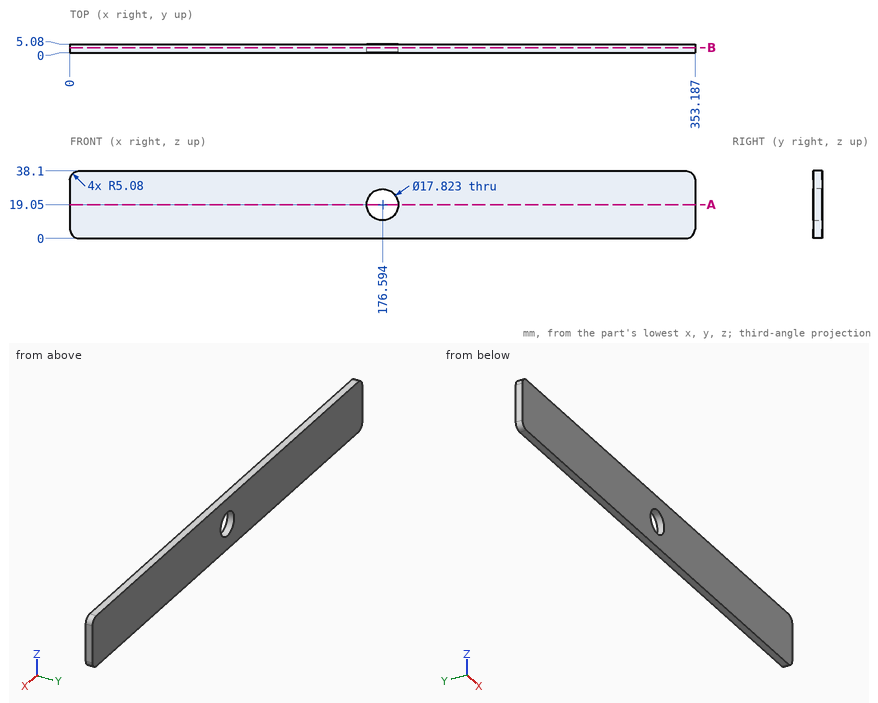
Check sheet for the drawn part. Datum: minimum x, y, z corner. Units: mm. Round coordinates to 2 decimals unless told otherwise and drop trailing zeros. Order: outer loops, then holes, each group sorted by start corner. A loop starts at its lowest first (then second) coordinate and runs counter-clockwise, first axis right, second up.
1. Thickness scan on L1, parallel to X at y = 2.95, z = 19.05 (1 decimal); L2, parallel to X at y = 4.8, z = 25 (1 decimal); L3, parallel to Z at x = 170, y = 0.45 (1 decimal). Record the ranges inside material, lowest first.
Final values:
L1: x = 0 to 167.7, 185.5 to 353.2
L2: x = 0 to 170, 183.2 to 353.2
L3: z = 0 to 13.1, 25 to 38.1
2. Section check B-B on y = 3.1. Record the cut outline in (x, z).
Final values:
outline: (0, 5.08) arc R5.08 ccw to (5.08, 0) - (348.11, 0) arc R5.08 ccw to (353.19, 5.08) - (353.19, 33.02) arc R5.08 ccw to (348.11, 38.1) - (5.08, 38.1) arc R5.08 ccw to (0, 33.02) - close; hole circle Ø17.82 at (176.59, 19.05)
3. Section check A-A on z = 19.05. Record the cut outline in (x, y) (1 decimal).
Final values:
outline: (0, 0) - (167.7, 0) - (167.7, 5.1) - (0, 5.1) - close; (185.5, 0) - (353.2, 0) - (353.2, 5.1) - (185.5, 5.1) - close
4. Go/stop test with a flat-tipped pin: P1, Ø10.5, axis at x = 176.59, z = 19.05, coming from the +Y side. Record where the tip stops, or that it passes through.
Final values:
P1: passes through
